CAD build for the part. Positions are in the model's coordinates, mm. Coordinates: 2 decimals unless noted, no trailing zeros. Loops run counter-clockwise (first coordinate to the right, second up) from the corner with the lowest first, then second, coordinate; pieces in that order, holes last. Notation, with made-up numbers: M -14.75,32.25 L 25.25,32.25 A17 cw 25.25,65.25 Z; hole C -5,-1 d1. An arc over 180 degrees is marked long. Answer as a JSON object with one key per item and string values. Group by question number.
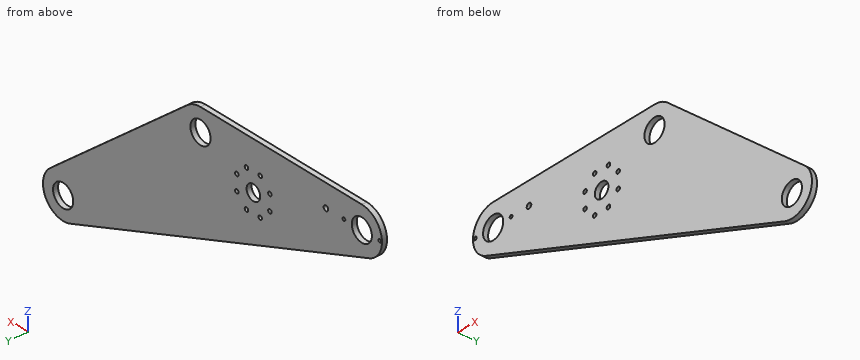
Autodesk Inventor part; units mm, degrees
ref_plane "YZ Plane" through (0, 0, 0) normal (1, 0, 0) x (0, 1, 0)
ref_plane "XZ Plane" through (0, 0, 0) normal (0, 1, 0) x (-1, 0, 0)
ref_plane "XY Plane" through (0, 0, 0) normal (0, 0, 1) x (1, 0, 0)
sketch "Sketch1" plane through (0, 0, 0) normal (0, 1, 0) x (-1, 0, 0)
  circle A0 centre (0, 0) radius 14.2875
  line L0 (0, 0) -> (228.6, 0) construction
  circle A1 centre (228.6, 0) radius 14.2875
  circle A2 centre (0, 0) radius 28.575 construction
  circle A3 centre (228.6, 0) radius 28.575 construction
  line L1 (228.6, -28.575) -> (0, -28.575)
  line L2 (0, 28.575) -> (228.6, 28.575)
  arc A4 (228.6, -28.575) -> (228.6, 28.575) centre (228.6, 0) ccw
  arc A5 (0, 28.575) -> (0, -28.575) centre (0, 0) ccw
  dimension "d0" = 28.575
  dimension "d1" = 228.6
  dimension "d5" = 57.15
extrude "Extrusion1" add sketch "Sketch1" along normal blind 6.35
sketch "Sketch3" plane through (0, 6.35, 0) normal (0, 1, 0) x (1, 0, 0)
  circle A0 centre (-228.6, 0) radius 14.2875 construction
  line L0 (0, 0) -> (-228.6, 0) construction
  circle A1 centre (0, 0) radius 14.2875 construction
  line L1 (0, 0) -> (194.5753, 163.2681) construction
  arc A2 (0, -28.575) -> (0, 28.575) centre (0, 0) ccw
  circle A3 centre (0, 0) radius 28.575
  circle A4 centre (194.5753, 163.2681) radius 28.575 construction
  circle A5 centre (194.5753, 163.2681) radius 14.2875
  circle A6 centre (0, 0) radius 14.2875
  line L2 (176.2076, 185.1578) -> (-18.3677, 21.8897)
  line L3 (212.9429, 141.3783) -> (18.3677, -21.8897)
  arc A7 (212.9429, 141.3783) -> (176.2076, 185.1578) centre (194.5753, 163.2681) ccw
  point P0 (0, 28.575)
  point P1 (18.3677, -21.8897)
  dimension "d12" = 254
  dimension "d13" = 140
extrude "Extrusion3" add sketch "Sketch3" against normal blind 6.35 contours A2 A3 L2 A7 L3
sketch "Sketch4" plane through (0, 6.35, 0) normal (0, 1, 0) x (1, 0, 0)
  circle A0 centre (-74.9321, 31.4901) radius 30 construction
  circle A1 centre (-74.9321, 31.4901) radius 25.4 construction
  circle A2 centre (-74.9321, 31.4901) radius 9.6012
  circle A3 centre (0, 0) radius 40.64 construction
  circle A4 centre (-74.9321, 31.4901) radius 40.64 construction
  line L0 (-84.6522, 8.0235) -> (-84.6522, 54.9566) construction
  line L1 (-84.6522, 54.9566) -> (-65.2119, 54.9566) construction
  line L2 (-65.2119, 54.9566) -> (-65.2119, 8.0235) construction
  line L3 (-65.2119, 8.0235) -> (-84.6522, 8.0235) construction
  circle A5 centre (-84.6522, 8.0235) radius 2.4892
  circle A6 centre (-65.2119, 8.0235) radius 2.4892
  circle A7 centre (-51.4655, 21.7699) radius 2.4892
  circle A8 centre (-51.4655, 41.2102) radius 2.4892
  line L4 (2.5406, 40.5605) -> (-2.5406, -40.5605) construction
  circle A9 centre (194.5753, 163.2681) radius 14.2875 construction
  line L5 (-74.9321, 31.4901) -> (194.5753, 163.2681) construction
  circle A10 centre (194.5753, 163.2681) radius 14.2875
  circle A11 centre (0, 0) radius 14.2875
  circle A12 centre (-228.6, 0) radius 14.2875
  line L6 (-10.4004, 28.575) -> (-228.6, 28.575)
  arc A13 (-228.6, 28.575) -> (-228.6, -28.575) centre (-228.6, 0) ccw
  line L7 (-228.6, -28.575) -> (0, -28.575)
  arc A14 (0, -28.575) -> (18.3677, -21.8897) centre (0, 0) ccw
  line L8 (18.3677, -21.8897) -> (212.9429, 141.3783)
  arc A15 (212.9429, 141.3783) -> (176.2076, 185.1578) centre (194.5753, 163.2681) ccw
  line L9 (176.2076, 185.1578) -> (-10.4004, 28.575)
  arc A16 (-228.6, 28.575) -> (-228.6, -28.575) centre (-228.6, 0) ccw
  circle A17 centre (0, 0) radius 50.8 construction
  arc A18 (-228.6, 28.575) -> (-228.6, -28.575) centre (-228.6, 0) ccw
  arc A19 (212.9429, 141.3783) -> (176.2076, 185.1578) centre (194.5753, 163.2681) ccw
  line L10 (-238.8857, 26.6596) -> (184.2896, 189.9277)
  circle A20 centre (-65.2119, 54.9566) radius 2.4892
  circle A21 centre (-84.6522, 54.9566) radius 2.4892
  circle A22 centre (-98.3986, 41.2102) radius 2.4892
  circle A23 centre (-98.3986, 21.7699) radius 2.4892
  point P0 (34.7284, 53.046)
  point P1 (38.9386, 55.4768)
  point P2 (-93.3302, 28.575)
  point P3 (-88.3521, 28.575)
  point P4 (-73.8899, 28.575)
  point P5 (-68.9118, 28.575)
  point P6 (-75.3508, 28.575)
  point P7 (-71.7292, 28.575)
  point P8 (-55.9105, 28.575)
  point P9 (-52.2889, 28.575)
  dimension "d16" = 60
  dimension "d17" = 50.8
  dimension "d18" = 19.2024
  dimension "d19" = 81.28
  dimension "d21" = 4.9784
  dimension "d24" = 360
  dimension "d26" = 299.9994
  dimension "d31" = 101.6
extrude "Extrusion7" cut sketch "Sketch4" against normal blind 6.35 contours A2 L6 | L6 A2 | A5 | A6 | A7 | A8 | A20 | A21 | A22 | A23
extrude "Extrusion8" add sketch "Sketch4" against normal blind 6.35 contours A2 L6 A13 L10 A15 L9
sketch "Sketch5" plane through (0, 6.35, 0) normal (0, 1, 0) x (1, 0, 0)
  line L0 (-238.8857, 26.6596) -> (184.2896, 189.9277)
  circle A0 centre (68.7646, 145.3562) radius 15.875
  point P0 (0, 0)
  dimension "d38" = 31.75
  dimension "d41" = 123.825
extrude "Extrusion9" [suppressed]
fillet "Fillet1" [suppressed]
sketch "Sketch6" plane through (0, 6.35, 0) normal (0, 1, 0) x (1, 0, 0)
  circle A0 centre (-228.6, 0) radius 14.2875 construction
  line L0 (-228.6, 0) -> (-177.8, 0) construction
  circle A1 centre (-177.8, 0) radius 3.2512
  point P0 (0, 0)
  dimension "d43" = 50.8
  dimension "d44" = 6.5024
extrude "Extrusion10" cut sketch "Sketch6" against normal blind 6.35
sketch "Sketch7" plane through (0, 6.35, 0) normal (0, 1, 0) x (1, 0, 0)
  circle A0 centre (-254, 0) radius 1.9812
  circle A1 centre (-203.2, 0) radius 1.9812
  line L0 (-203.2, 0) -> (-254, 0) construction
  circle A2 centre (-228.6, 0) radius 14.2875 construction
  point P0 (0, 0)
  dimension "d47" = 50.8
  dimension "d48" = 3.9624
extrude "Extrusion11" cut sketch "Sketch7" against normal blind 6.35
thread "Thread1"
thread "Thread2"
properties part number "CORL_006_SmallPlate" material "Polycarbonate, Clear"
Item 1: Slice it at D-D, the plane x = 148. Write the cut outline in (y, z).
Item 2: Slice it at B-B, the plane y = 1.5. Count the separate pieces of the cut face and the enclosed holes in it, then the cut area to 3 significant figures.
Item 3: Slice it at A-A, the plane x = -77. Write the cut outline in (y, z) (3 decimals).
Item 4: Drill centre lines: L1, parallel to Z at x = 195, y = 4.25; L2, parallel to X at y = 3.25, z = -25; L3, parallel to Z at x = -74.5, y = 3.5 (3 decimals). Where is each one in solid material? Low to high. Write a range as from..to.
Item 5: Slice it at C-C, the plane z = -95. Write the cut outline in (x, y), then the cut area to 3 significant figures.
Item 6: Pin check, flat tip, straight feed: pin 1 (8 mm diameter, centred on x = -51.47, z = -41.21, fed in from -Y). Stop position of the tip, or through.
Computed:
{
 "1": {"outline": "M 0,-175.93 L 6.35,-175.93 L 6.35,-86.88 L 0,-86.88 Z"},
 "2": {"separate pieces": "1", "enclosed holes": "15", "area": "45,600 mm2"},
 "3": {"outline": "M 0,-89.118 L 6.35,-89.118 L 6.35,-40.866 L 0,-40.866 Z; M 0,-22.114 L 6.35,-22.114 L 6.35,28.575 L 0,28.575 Z"},
 "4": {"L1": "-191.84..-177.55, -148.99..-126.32", "L2": "-242.44..-82.01, -67.86..74.25", "L3": "-90.082..-41.082, -21.899..28.575"},
 "5": {"outline": "M -61.75,0 L 157.67,0 L 157.67,6.35 L -61.75,6.35 Z", "area": "1,390 mm2"},
 "6": {"pin 1": "y = 0"}
}
